```python
from build123d import *

# Parameters (mm, degrees)
BOSS_EXTRUDE1_DEPTH = 20
CUT_EXTRUDE1_DEPTH  = 46.961940777
FILLET1_R           = 1
FILLET2_R           = 1
FILLET3_R           = 1


with BuildPart() as part:
    # Sketch1 → Boss-Extrude1 (new body)
    with BuildSketch(Plane.XY):
        with BuildLine():
            Line((-19.5, 0), (-16.5, 0))
            ThreePointArc((-16.5, 0), (-11.66726189, 11.66726189), (0, 16.5))
            Line((0, 16.5), (0, 34.5))
            ThreePointArc((0, 34.5), (-0.585786438, 35.914213562), (-2, 36.5))
            Line((-2, 36.5), (-13, 36.5))
            ThreePointArc((-13, 36.5), (-14.414213562, 35.914213562), (-15, 34.5))
            Line((-15, 34.5), (-15, 15.660459763))
            ThreePointArc((-15, 15.660459763), (-15.388918825, 12.89873591), (-16.525423729, 10.351829335))
            ThreePointArc((-16.525423729, 10.351829335), (-18.741608292, 5.385361515), (-19.5, 0))
        make_face()
    extrude(amount=BOSS_EXTRUDE1_DEPTH)

    # Sketch2 → Cut-Extrude1 (cut, through all)
    with BuildSketch(Plane(origin=(0, 0, 0), x_dir=(0, 0, -1), z_dir=(1, 0, 0))):
        with BuildLine():
            Line((-11.5, 19.0873018), (-8.5, 19.0873018))
            Line((-8.5, 19.0873018), (-8.5, 20.5873018))
            ThreePointArc((-8.5, 20.5873018), (-10, 32.6), (-11.5, 20.5873018))
            Line((-11.5, 20.5873018), (-11.5, 19.0873018))
        make_face()
    extrude(amount=-CUT_EXTRUDE1_DEPTH, mode=Mode.SUBTRACT)

    # Fillet1
    fillet1_edges = [part.edges().sort_by_distance(p)[0] for p in [
        (-15, 19.0873018, 10),
        (0, 19.0873018, 10),
    ]]
    fillet(fillet1_edges, radius=FILLET1_R)

    # Fillet2
    fillet2_edges = [part.edges().sort_by_distance(p)[0] for p in [
        (-15, 32.6, 10),
        (0, 32.6, 10),
    ]]
    fillet(fillet2_edges, radius=FILLET2_R)

    # Fillet3
    fillet3_edges = [part.edges().sort_by_distance(p)[0] for p in [
        (-11.66726189, 11.66726189, 20),
        (-0.585786438, 35.914213562, 0),
        (0, 25.5, 0),
        (-11.66726189, 11.66726189, 0),
        (-18, 0, 0),
        (-18.741608292, 5.385361515, 0),
        (0, 25.5, 20),
        (-0.585786438, 35.914213562, 20),
        (-7.5, 36.5, 20),
        (-14.414213562, 35.914213562, 20),
        (-15, 25.080229882, 20),
        (-15.388918825, 12.89873591, 20),
        (-18.741608292, 5.385361515, 20),
        (-18, 0, 20),
        (-15.388918825, 12.89873591, 0),
        (-15, 25.080229882, 0),
        (-14.414213562, 35.914213562, 0),
        (-7.5, 36.5, 0),
    ]]
    fillet(fillet3_edges, radius=FILLET3_R)


solid = part.part
```
Source: CAD feature listing. Evaluate the final solid. Frame: model axes, mm. A direction names the side the tool comes from. Give positions to 0.01 mm unless a question says otherwise; leave off trailing zeros. Order: outer loops, then holes, each group sorted by start corner. A loop starts at its lowest first (then second) coordinate and runs counter-clockwise, first axis right, second up.
(1) Pull-direction query (Z, two-part tool) for faces 6 (the face through (-7, 20, 11.5)), 7 (the face through (-8, 26, 0)), 8 (the face through (0, 19, 12)); classes: +Z half, -Z half, draft (parallel to the pull), parting line (faces both ways), or undercut.
(2) Section query A-A (z = 10). Return the cut outline in (x, y).
(3) Material intervals for line 1 along Z through (x, y) = (-9.5, 26.5); line 2 along X through (y, z) = (27.5, 2.5); line 3 along Z through (x, y) = (-14.25, 21), sorted ascending.
(4) Access query for faces 1 (the face through (-14.7, 18.8, 10)), 2 (the face through (-7, 19.087, 10)), 3 (the face through (-14.715, 24.948, 19.699)), 4 (the face through (-0.3, 18.8, 10)), 5 (the face through (-14.715, 24.948, 0.301)). Directions: +Z, -Z, +X, -X, +Y, -Y. A direction counts if a zero-diameter tool reaches every point of the face in a straight line with its end or side. Return the directions, or none.
(5) Contact query for flat-ended pins moving along their axis: P1, Ø10, axis at y = 7, z = 6.5, coming from the -X side; P2, Ø6, axis at y = 32.5, z = 16.5, coming from the -X side. Output: stop coordinate, or through.
Outcome:
1. face 6: undercut
1. face 7: -Z half
1. face 8: draft
2. outline: (-19.5, 0) - (-16.5, 0) arc R16.5 cw to (0, 16.5) - (0, 18.09) arc R1 ccw to (-1, 19.09) - (-14, 19.09) arc R1 ccw to (-15, 18.09) - (-15, 15.66) arc R10 cw to (-16.53, 10.35) arc R19.5 ccw to start; (-15, 33.6) arc R1 ccw to (-14, 32.6) - (-1, 32.6) arc R1 ccw to (0, 33.6) - (0, 34.5) arc R2 ccw to (-2, 36.5) - (-13, 36.5) arc R2 ccw to (-15, 34.5) - close
3. line 1: z = 0 to 3.9, 16.1 to 20
3. line 2: x = -15 to 0
3. line 3: z = 0.03 to 7.29, 12.71 to 19.97
4. face 1: -X
4. face 2: +X, -X
4. face 3: +Z, -X, +Y
4. face 4: +X
4. face 5: -Z, -X, +Y
5. P1: stops at x = -19.4
5. P2: stops at x = -15
